```python
from build123d import *

# Parameters (mm, degrees)
SKETCH1_R           = 6.6
SKETCH1_W           = 20.2
SKETCH1_H           = 40.2
BASE_PLATE_DEPTH    = 4
FILLET1_R           = 1
FILLET2_R           = 2
SKETCH2_R           = 1.7
CUT_EXTRUDE1_DEPTH  = 78.256779638
SKETCH3_W           = 4
SKETCH3_H           = 40.2
BOSS_EXTRUDE1_DEPTH = 28.2
CUT_EXTRUDE2_DEPTH  = 78.256779638
FILLET3_R           = 1


with BuildPart() as part:
    # Sketch1 → Base Plate (new body)
    with BuildSketch(Plane.XY):
        with BuildLine():
            Line((-4.9, -75), (4.9, -75))
            ThreePointArc((4.9, -75), (14.233809512, -71.133809512), (18.1, -61.8))
            Line((18.1, -61.8), (18.1, 75))
            Line((18.1, 75), (-18.1, 75))
            Line((-18.1, 75), (-18.1, -61.8))
            ThreePointArc((-18.1, -61.8), (-14.233809512, -71.133809512), (-4.9, -75))
        make_face()
        with Locations((0, -50.1)):
            Circle(SKETCH1_R, mode=Mode.SUBTRACT)
        Polygon((-10.1, 28.1), (4.1, 28.1), (-10.1, 67), align=None, mode=Mode.SUBTRACT)
        Rectangle(SKETCH1_W, SKETCH1_H, mode=Mode.SUBTRACT)
        Polygon((10.1, 67), (-4.1, 67), (10.1, 28.1), align=None, mode=Mode.SUBTRACT)
    extrude(amount=BASE_PLATE_DEPTH)

    # Fillet1
    fillet1_edges = [part.edges().sort_by_distance(p)[0] for p in [
        (10.1, 28.1, 2),
        (10.1, 67, 2),
        (-4.1, 67, 2),
        (-10.1, 67, 2),
        (-10.1, 28.1, 2),
        (4.1, 28.1, 2),
    ]]
    fillet(fillet1_edges, radius=FILLET1_R)

    # Fillet2
    fillet2_edges = [part.edges().sort_by_distance(p)[0] for p in [
        (-18.1, 75, 2),
        (18.1, 75, 2),
    ]]
    fillet(fillet2_edges, radius=FILLET2_R)

    # Sketch2 → Cut-Extrude1 (cut, through all)
    with BuildSketch(Plane.XY.offset(4)):
        with Locations((5, 24.75)):
            Circle(SKETCH2_R)
        with Locations((-5, 24.75)):
            Circle(SKETCH2_R)
        with Locations(Location((-5, -24.75, 0), (0, 0, 180))):
            Circle(SKETCH2_R)
        with Locations(Location((5, -24.75, 0), (0, 0, 180))):
            Circle(SKETCH2_R)
        with Locations((13.4, 24.75)):
            Circle(SKETCH2_R)
        with Locations(Location((-13.4, 24.75, 0), (0, 0, 180))):
            Circle(SKETCH2_R)
        with Locations(Location((13.4, -24.75, 0), (0, 0, 180))):
            Circle(SKETCH2_R)
        with Locations((-13.4, -24.75)):
            Circle(SKETCH2_R)
        with Locations((13.4, 70.3)):
            Circle(SKETCH2_R)
        with Locations(Location((-13.4, 70.3, 0), (0, 0, 180))):
            Circle(SKETCH2_R)
        with Locations((0, -69.3)):
            Circle(SKETCH2_R)
    extrude(amount=-CUT_EXTRUDE1_DEPTH, mode=Mode.SUBTRACT)

    # Sketch3 → Boss-Extrude1 (add, through all)
    with BuildSketch(Plane.ZY.offset(-10.1)):
        with Locations((2, 0)):
            Rectangle(SKETCH3_W, SKETCH3_H)
    extrude(amount=BOSS_EXTRUDE1_DEPTH)

    # Sketch4 → Cut-Extrude2 (cut, through all)
    with BuildSketch(Plane.XY.offset(4)):
        Polygon((-10.1, 20.1), (-10.1, -20.1), (3.9, -20.1), align=None)
        Polygon((-3.9, 20.1), (10.1, 20.1), (10.1, -20.1), align=None)
    extrude(amount=-CUT_EXTRUDE2_DEPTH, mode=Mode.SUBTRACT)

    # Fillet3
    fillet3_edges = [part.edges().sort_by_distance(p)[0] for p in [
        (10.1, -20.1, 2),
        (-3.9, 20.1, 2),
        (10.1, 20.1, 2),
        (-10.1, 20.1, 2),
        (3.9, -20.1, 2),
        (-10.1, -20.1, 2),
    ]]
    fillet(fillet3_edges, radius=FILLET3_R)


solid = part.part
```
Geometry: final body of the model. Coordinates: model frame, mm. A direction names the side the tool comes from. Round coordinates to 2 decimals unless told otherwise and drop trailing zeros. Order: outer loops, then holes, each group sorted by start corner. A loop starts at its lowest first (then second) coordinate and runs counter-clockwise, first axis right, second up. Notation, with made-up numbers: M 27,10 L 71,10 A8 cw 71,20 Z; hole C 67.5,-35 d6. An arc over 180 degrees is marked long. Use one line per item in the form item = value. Start each with the question number.
Q1. Cut plane B-B (y = -50.1). Return loops of the section in (x, z).
Q2. Cut plane C-C (y = 24.75). Return loops of the section in (x, z), and give its area (3 significant figures).
Q3. Material intervals for line 1 (X direction, y = 70.3, z = 2.85); line 2 (Y direction, x = -9, z = 0.9); line 3 (Y direction, x = -13, z = 1.85), sorted ascending. Write a range as [from, to].
Q4. Cut plane A-A (y = 70.3). Return loops of the section in (x, z).
Q5. Mould query, pull axis Y, two halves, no side actions, for faces 3 (the face through (0, 1, 0)), 4 (the face through (0, 75, 2)), 5 (the face through (-2.28, -2.36, 2.03)), 6 (the face through (3, 67, 2)). Classes: +Y half, -Y half, draft (parallel to the pull), parting line (faces both ways), or undercut.
Q6. Cut plane D-D (x = -13.4). Return loops of the section in (y, z).
Q7. Pin query (flat end, axial travel): pin 1 Ø1.5 at (x, z) = (6, 2) entering from -Y; pin 2 Ø3 at (x, y) = (13.4, 24.75) entering from +Z. Return the tip coordinate at first contact, or that it passes through.
Q8. Access query for faces 1 (the face through (-14.336, -71.031, 1.972)), 2 (the face through (-2.193, 45.339, 1.972)). Directions: +Z, -Z, +X, -X, +Y, -Y. A direction counts if a zero-diameter tool reaches every point of the face in a straight line with its end or side. Return the directions, or none.
Geometry results:
q1.outline = M -18.1,0 L -6.6,0 L -6.6,4 L -18.1,4 Z; M 6.6,0 L 18.1,0 L 18.1,4 L 6.6,4 Z
q2.outline = M -18.1,0 L -15.1,0 L -15.1,4 L -18.1,4 Z; M -11.7,0 L -6.7,0 L -6.7,4 L -11.7,4 Z; M -3.3,0 L 3.3,0 L 3.3,4 L -3.3,4 Z; M 6.7,0 L 11.7,0 L 11.7,4 L 6.7,4 Z; M 15.1,0 L 18.1,0 L 18.1,4 L 15.1,4 Z
q2.area = 90.4 mm^2
q3.line_1 = [-18.1, -15.1], [-11.7, 11.7], [15.1, 18.1]
q3.line_2 = [-74.35, -20.1], [15.18, 28.1], [62.34, 75]
q3.line_3 = [-72.22, -26.4], [-23.1, 23.1], [26.4, 68.65], [71.95, 75]
q4.outline = M -18.1,0 L -15.1,0 L -15.1,4 L -18.1,4 Z; M -11.7,0 L 11.7,0 L 11.7,4 L -11.7,4 Z; M 15.1,0 L 18.1,0 L 18.1,4 L 15.1,4 Z
q5.face_3 = draft
q5.face_4 = +Y half
q5.face_5 = undercut
q5.face_6 = undercut
q6.outline = M -71.9,0 L -26.45,0 L -26.45,4 L -71.9,4 Z; M -23.05,0 L 23.05,0 L 23.05,4 L -23.05,4 Z; M 26.45,0 L 68.6,0 L 68.6,4 L 26.45,4 Z; M 72,0 L 75,0 L 75,4 L 72,4 Z
q7.pin_1 = -75
q7.pin_2 = through
q8.face_1 = +Z, -Z, -X, -Y
q8.face_2 = +Z, -Z
